For this review, take the finished solid that the model builds, in its own axes (mm). Face numbers are marked on the shaded views. A direction names the side the tool comes from. Give positions to 0.01 mm unless a question says otherwise; leave off trailing zeros. Loops run counter-clockwise (first coordinate to the right, second up) from the corner with the lowest first, then second, coordinate; pieces in that order, holes last.
```python
from build123d import *

# Parameters (mm, degrees)
SKETCH1_R                = 4.7498
EXTRUDE1_DEPTH           = 11.43
SKETCH3_R                = 4.7498
CUT_EXTRUDE1_DEPTH       = 1.905
CHAMFER1_SIZE            = 0.635
CHAMFER1_OF_MIRROR1_SIZE = 0.635


with BuildPart() as part:
    # Sketch1 → Extrude1 (new body)
    with BuildSketch(Plane.XY):
        with Locations((22.45995, 0)):
            Circle(SKETCH1_R)
    extrude1 = extrude(amount=EXTRUDE1_DEPTH)

    # Sketch2 → Cut-Revolve1 (revolve, cut)
    with BuildSketch(Plane(origin=(0, 0, 0), x_dir=(-1, 0, 0), z_dir=(0, 1, 0))):
        Polygon((-18.77695, 5.08), (-16.87195, 6.985), (-16.87195, 3.175), align=None)
    cut_revolve1 = revolve(axis=Axis((22.45995, 0, 11.43), (0, 0, -1)), mode=Mode.SUBTRACT)

    # Sketch3 → Cut-Extrude1 (cut)
    with BuildSketch(Plane(origin=(0, 0, 0), x_dir=(-1, 0, 0), z_dir=(0, 0, -1))):
        with Locations((-22.45995, 0)):
            Circle(SKETCH3_R)
    cut_extrude1 = extrude(amount=-CUT_EXTRUDE1_DEPTH, mode=Mode.SUBTRACT)

    # Chamfer1
    chamfer1_edges = [part.edges().sort_by_distance(p)[0] for p in [
        (17.71015, 0, 1.905),
    ]]
    chamfer(chamfer1_edges, length=CHAMFER1_SIZE)

    # Mirror1: Extrude1, Cut-Revolve1, Cut-Extrude1 across plane
    add(extrude1.mirror(Plane(origin=(28.80995, -13.97, 11.43), x_dir=(1, 0, 0), z_dir=(0, 0, -1))))
    add(cut_revolve1.mirror(Plane(origin=(28.80995, -13.97, 11.43), x_dir=(1, 0, 0), z_dir=(0, 0, -1))), mode=Mode.SUBTRACT)
    add(cut_extrude1.mirror(Plane(origin=(28.80995, -13.97, 11.43), x_dir=(1, 0, 0), z_dir=(0, 0, -1))), mode=Mode.SUBTRACT)

    # Chamfer1 of Mirror1
    chamfer1_of_mirror1_edges = [part.edges().sort_by_distance(p)[0] for p in [
        (17.71015, 0, 20.955),
    ]]
    chamfer(chamfer1_of_mirror1_edges, length=CHAMFER1_OF_MIRROR1_SIZE)


solid = part.part
```
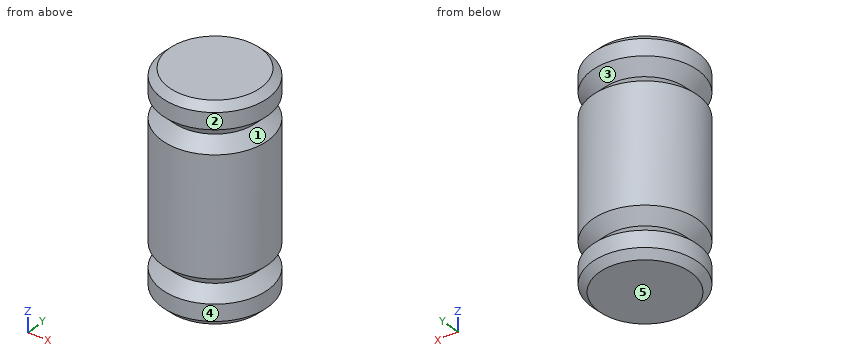
Q1. Consider section A-A on y = 3.75. Count the separate pieces of the cut face and the enclosed holes in it, plus the area to 3 significant figures.
Answers:
separate pieces: 3
enclosed holes: 0
area: 99.9 mm2
Q2. Mouldability with a two-part tool opening along Z and no side actions: class the marked faces 3, 4 and 5 as +Z half, -Z half, draft (parallel to the pull), parting line (faces both ways), or undercut.
Answers:
face 3: undercut
face 4: draft
face 5: -Z half
Q3. For probe 1 along Z at (x, y) = (24, 4.25); probe 2 along Z at (x, y) = (21.5, 4.25); probe 3 along X at (y, z) = (4, 3.5), list the stretches that pass through material, from the lowest coordinate up.
Answers:
probe 1: z = 2.31 to 4.24, 5.92 to 16.94, 18.62 to 20.55
probe 2: z = 2.15 to 4.41, 5.75 to 17.11, 18.45 to 20.71
probe 3: x = 19.9 to 25.02
Q4. Machinability: for the marked faces 1 and 2, which of the approach directions +Z, -Z, +X, -X, +Y, -Y give a long, thin tool a straight path to every point of the face, cutting with its end or side? Answer none if there is none.
Answers:
face 1: none
face 2: +Z, -Z
Q5. Consider section D-D on z = 5.5. Give the boundary of the cut face in (x, y).
Answers:
outline: circle Ø8.21 at (22.46, 0)
Q6. Consider section B-B on z = 7.75. Give the boundary of the cut face in (x, y), plus the area to 3 significant figures.
Answers:
outline: circle Ø9.5 at (22.46, 0)
area: 70.9 mm2
Q7. For pin 1 Ø1 at (y, z) = (-1, 5.5) entering from -X; pin 2 Ø1 at (x, z) = (19.5, 9.5) entering from +Y; pin 3 Ø2 at (y, z) = (3.5, 7) entering from -X, all flat-tipped, find the tip position at first contact; note any pin that passes through.
Answers:
pin 1: stops at x = 17.96
pin 2: stops at y = 4.06
pin 3: stops at x = 18.42
Q8. Consider section C-C on y = 0. Give the boundary of the cut face in (x, z) (3 decimals).
Answers:
outline: (17.71, 2.54) - (18.345, 1.905) - (26.575, 1.905) - (27.21, 2.54) - (27.21, 4.013) - (26.143, 5.08) - (27.21, 6.147) - (27.21, 16.713) - (26.143, 17.78) - (27.21, 18.847) - (27.21, 20.32) - (26.575, 20.955) - (18.345, 20.955) - (17.71, 20.32) - (17.71, 18.847) - (18.777, 17.78) - (17.71, 16.713) - (17.71, 6.147) - (18.777, 5.08) - (17.71, 4.013) - close
